Here's how the part is built. I have some questions about the finished solid (model axes, mm). Face numbers are marked on the shaded views. A direction names the side the tool comes from. Coordinates: 2 decimals unless noted, no trailing zeros. Order: outer loops, then holes, each group sorted by start corner. A loop starts at its lowest first (then second) coordinate and runs counter-clockwise, first axis right, second up. Notation, with made-up numbers: (42, 15) - (55, 15) arc R26 cw to (55, 41) - close; hole circle Ø10 at (45, -25.75). An arc over 180 degrees is marked (long way). Answer in a Markdown table with one row per item. Add a question column.
Item 1: I want a section at B-B (z = 35). Please give me the cut outline in (x, y).
Item 2: On a 3-axis mill with a long thin cutter (end or side, diameter ignored), from which of +Z, -Z, +X, -X, +Y, -Y can I reach the whole of each face in a straight line? I mean the marked faces 1, 2, 3 and 4. Say none if no direction works.
Item 3: I want a section at C-C (y = 24.5). Please give me the cut outline in (x, z).
Item 4: I want a section at D-D (x = 12.5). Please give me the cut outline in (y, z).
Item 5: If I drill on line 1 along X through (y, z) = (3.25, 27); line 2 along Z through (x, y) = (26.5, 22); line 3 along Z through (x, y) = (8.5, 2), over which ranges is the centre line in solid material (lowest first)? Write a range as from..to.
Item 6: Thinking about a two-plate mould opening in Z: for the marked faces 5, 6 and 7, which applies, +Z half, -Z half, draft (parallel to the pull), parting line (faces both ways), or undercut?
Item 7: I want a section at A-A (y = 15.5). Please give me the cut outline in (x, z).
Item 8: Will these pins go through, and if not, where does the flat tip stop? pin 1 Ø8.5 at (y, z) = (14.5, 12) entering from +X; pin 2 Ø1.3 at (x, z) = (8.5, 28) entering from -Y; pin 3 Ø3 at (x, z) = (16.5, 36) entering from -Y.
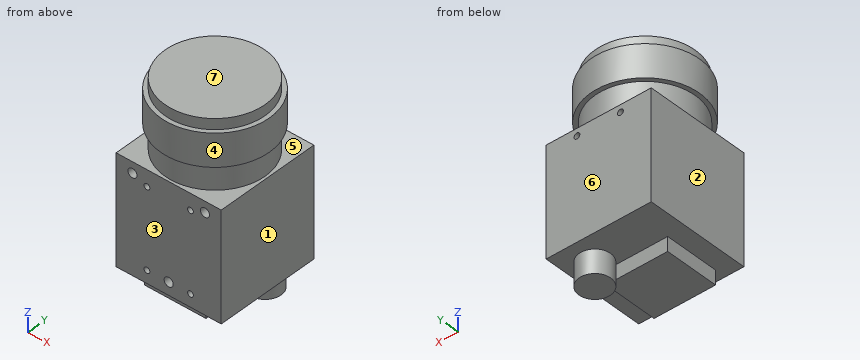
```python
from build123d import *

# Parameters (mm, degrees)
SKETCH1_W                 = 29
SKETCH1_H                 = 29
BOSS_EXTRUDE1_DEPTH       = 30
SKETCH2_R                 = 13.8303
BOSS_EXTRUDE2_DEPTH       = 18.8722
M2X0_4_TAPPED_HOLE1_D     = 1.6
M2X0_4_TAPPED_HOLE1_DEPTH = 8.31088
M2X0_4_TAPPED_HOLE1_TIP   = 0.480688495
M2X0_4_TAPPED_HOLE2_D     = 1.6
M2X0_4_TAPPED_HOLE2_DEPTH = 8.31088
M2X0_4_TAPPED_HOLE2_TIP   = 0.480688495
M3X0_5_TAPPED_HOLE1_D     = 2.5
M3X0_5_TAPPED_HOLE1_DEPTH = 7.50062
M3X0_5_TAPPED_HOLE1_TIP   = 0.751075774
SKETCH15_R                = 4.3561
BOSS_EXTRUDE4_DEPTH       = 3.937
SKETCH15_7_R              = 4.3561
BOSS_EXTRUDE5_DEPTH       = 6.4516
BOSS_EXTRUDE6_START       = 6.9342
SKETCH2_5_R               = 14.9987
BOSS_EXTRUDE6_DEPTH       = 9.017


with BuildPart() as part:
    # Sketch1 → Boss-Extrude1 (new body)
    with BuildSketch(Plane.XY):
        with Locations((14.5, 14.5)):
            Rectangle(SKETCH1_W, SKETCH1_H)
    extrude(amount=BOSS_EXTRUDE1_DEPTH)

    # Sketch2 → Boss-Extrude2 (add)
    with BuildSketch(Plane.XY.offset(30)):
        with Locations((14.5, 14.5)):
            Circle(SKETCH2_R)
    extrude(amount=BOSS_EXTRUDE2_DEPTH)

    # M2x0.4 Tapped Hole1
    with Locations(Plane(origin=(0, 0, 0), x_dir=(-1, 0, 0), z_dir=(0, -1, 0))):
        with Locations((-20.5, -3.5), (-20.5, -25.5), (-8.5, -3.5), (-8.5, -25.5)):
            Hole(M2X0_4_TAPPED_HOLE1_D / 2, depth=M2X0_4_TAPPED_HOLE1_DEPTH)
            with Locations((0, 0, -(M2X0_4_TAPPED_HOLE1_DEPTH + M2X0_4_TAPPED_HOLE1_TIP / 2))):  # 118° drill point
                Cone(0, M2X0_4_TAPPED_HOLE1_D / 2, M2X0_4_TAPPED_HOLE1_TIP, mode=Mode.SUBTRACT)

    # M2x0.4 Tapped Hole2
    with Locations(Plane(origin=(0, 29, 0), x_dir=(1, 0, 0), z_dir=(0, 1, 0))):
        with Locations((20.5, -28), (8.5, -28)):
            Hole(M2X0_4_TAPPED_HOLE2_D / 2, depth=M2X0_4_TAPPED_HOLE2_DEPTH)
            with Locations((0, 0, -(M2X0_4_TAPPED_HOLE2_DEPTH + M2X0_4_TAPPED_HOLE2_TIP / 2))):  # 118° drill point
                Cone(0, M2X0_4_TAPPED_HOLE2_D / 2, M2X0_4_TAPPED_HOLE2_TIP, mode=Mode.SUBTRACT)

    # M3x0.5 Tapped Hole1
    with Locations(Plane(origin=(0, 0, 0), x_dir=(-1, 0, 0), z_dir=(0, -1, 0))):
        with Locations((-14.5, -3.5), (-4.5, -27), (-24.5, -27)):
            Hole(M3X0_5_TAPPED_HOLE1_D / 2, depth=M3X0_5_TAPPED_HOLE1_DEPTH)
            with Locations((0, 0, -(M3X0_5_TAPPED_HOLE1_DEPTH + M3X0_5_TAPPED_HOLE1_TIP / 2))):  # 118° drill point
                Cone(0, M3X0_5_TAPPED_HOLE1_D / 2, M3X0_5_TAPPED_HOLE1_TIP, mode=Mode.SUBTRACT)

    # Sketch15 → Boss-Extrude4 (add)
    with BuildSketch(Plane(origin=(0, 0, 0), x_dir=(-1, 0, 0), z_dir=(0, 0, -1))):
        with BuildLine():
            Line((-5.1308, 18.034), (-19.572374024, 18.034))
            ThreePointArc((-19.572374024, 18.034), (-20.772304505, 17.433725495), (-22.098, 17.2271))
            Line((-22.098, 17.2271), (-22.098, 3.048))
            Line((-22.098, 3.048), (-5.1308, 3.048))
            Line((-5.1308, 3.048), (-5.1308, 18.034))
        make_face()
        with Locations((-22.098, 21.5832)):
            Circle(SKETCH15_R)
    extrude(amount=BOSS_EXTRUDE4_DEPTH)

    # Sketch15_7 → Boss-Extrude5 (add)
    with BuildSketch(Plane(origin=(0, 0, 0), x_dir=(-1, 0, 0), z_dir=(0, 0, -1))):
        with Locations((-22.098, 21.5832)):
            Circle(SKETCH15_7_R)
    extrude(amount=BOSS_EXTRUDE5_DEPTH)

    # Sketch2_5 → Boss-Extrude6 (add)
    with BuildSketch(Plane.XY.offset(30).offset(BOSS_EXTRUDE6_START)):
        with Locations((14.5, 14.5)):
            Circle(SKETCH2_5_R)
    extrude(amount=BOSS_EXTRUDE6_DEPTH)


solid = part.part
```
Values follow:
| question | item | result |
|---|---|---|
| 1 | outline | circle Ø27.66 at (14.5, 14.5) |
| 2 | face 1 | -Z, +X, +Y, -Y |
| 2 | face 2 | -Z, -X, +Y, -Y |
| 2 | face 3 | -Z, +X, -X, -Y |
| 2 | face 4 | +Z |
| 3 | outline | (0, 0) - (18.86, 0) - (18.86, -6.45) - (25.33, -6.45) - (25.33, 0) - (29, 0) - (29, 30) - (24.05, 30) - (24.05, 36.93) - (25.68, 36.93) - (25.68, 45.95) - (24.05, 45.95) - (24.05, 48.87) - (4.95, 48.87) - (4.95, 45.95) - (3.32, 45.95) - (3.32, 36.93) - (4.95, 36.93) - (4.95, 30) - (0, 30) - close; hole circle Ø1.6 at (8.5, 28); hole circle Ø1.6 at (20.5, 28) |
| 4 | outline | (-0.36, 36.93) - (0.82, 36.93) - (0.82, 30) - (0, 30) - (0, 0) - (3.05, 0) - (3.05, -3.94) - (18.03, -3.94) - (18.03, 0) - (29, 0) - (29, 30) - (28.18, 30) - (28.18, 36.93) - (29.36, 36.93) - (29.36, 45.95) - (28.18, 45.95) - (28.18, 48.87) - (0.82, 48.87) - (0.82, 45.95) - (-0.36, 45.95) - close |
| 5 | line 1 | x = 0..3.25, 5.75..23.25, 25.75..29 |
| 5 | line 2 | z = 0..30, 36.93..45.95 |
| 5 | line 3 | z = 0..2.7, 4.3..24.7, 26.3..30, 36.93..45.95 |
| 6 | face 5 | undercut |
| 6 | face 6 | draft |
| 6 | face 7 | +Z half |
| 7 | outline | (-0.47, 36.93) - (0.71, 36.93) - (0.71, 30) - (0, 30) - (0, 0) - (5.13, 0) - (5.13, -3.94) - (22.1, -3.94) - (22.1, 0) - (29, 0) - (29, 30) - (28.29, 30) - (28.29, 36.93) - (29.47, 36.93) - (29.47, 45.95) - (28.29, 45.95) - (28.29, 48.87) - (0.71, 48.87) - (0.71, 45.95) - (-0.47, 45.95) - close |
| 8 | pin 1 | stops at x = 29 |
| 8 | pin 2 | stops at y = 0 |
| 8 | pin 3 | stops at y = -0.48 |
